Geometry check sheet. Reference: the model listing, model coordinates, mm. A direction names the side the tool comes from. Give positions to 0.01 mm unless a question says otherwise; leave off trailing zeros. Loops run counter-clockwise (first coordinate to the right, second up) from the corner with the lowest first, then second, coordinate; pieces in that order, holes last. Notation, with made-up numbers: (61.25, 18.5) -> (103.25, 18.5) arc R30 cw to (103.25, 48.5) -> close; hole circle Ø5 at (-18, 17). An arc over 180 degrees is marked (long way). Write item = value, one per line. Start each with the question number.
```python
from build123d import *

# Parameters (mm, degrees)
BOSS_EXTRU_1_DEPTH      = 1
ENL_V_MAT_EXTRU_1_DEPTH = 1
BOSS_EXTRU_2_DEPTH      = 5
ESQUISSE4_W             = 8.8
ESQUISSE4_H             = 7.4
ENL_V_MAT_EXTRU_2_DEPTH = 0.5


with BuildPart() as part:
    # Esquisse1 → Boss.-Extru.1 (new body)
    with BuildSketch(Plane.XY):
        with BuildLine():
            Line((-19.325920559, 52.160343492), (-47.644494554, 40.430406076))
            ThreePointArc((-47.644494554, 40.430406076), (-48.617764601, 39.780087822), (-49.268082855, 38.806817776))
            Line((-49.268082855, 38.806817776), (-60.99802027, 10.488243781))
            ThreePointArc((-60.99802027, 10.488243781), (-61.226381673, 9.340193484), (-60.99802027, 8.192143187))
            Line((-60.99802027, 8.192143187), (-49.268082855, -20.126430808))
            ThreePointArc((-49.268082855, -20.126430808), (-48.617764601, -21.099700855), (-47.644494554, -21.750019109))
            Line((-47.644494554, -21.750019109), (-19.325920559, -33.479956525))
            ThreePointArc((-19.325920559, -33.479956525), (-18.177870262, -33.708317927), (-17.029819965, -33.479956525))
            Line((-17.029819965, -33.479956525), (11.28875403, -21.750019109))
            ThreePointArc((11.28875403, -21.750019109), (12.262024077, -21.099700855), (12.912342331, -20.126430808))
            Line((12.912342331, -20.126430808), (24.642279746, 8.192143187))
            ThreePointArc((24.642279746, 8.192143187), (24.870641149, 9.340193484), (24.642279746, 10.488243781))
            Line((24.642279746, 10.488243781), (12.912342331, 38.806817776))
            ThreePointArc((12.912342331, 38.806817776), (12.262024077, 39.780087822), (11.28875403, 40.430406076))
            Line((11.28875403, 40.430406076), (-17.029819965, 52.160343492))
            ThreePointArc((-17.029819965, 52.160343492), (-18.177870262, 52.388704894), (-19.325920559, 52.160343492))
        make_face()
    extrude(amount=BOSS_EXTRU_1_DEPTH)

    # Esquisse2 → Enlèv. mat.-Extru.1 (cut)
    with BuildSketch(Plane.XY.offset(1)):
        with BuildLine():
            Line((-21.671668776, 13.7151444), (-17.371668776, 13.7151444))
            ThreePointArc((-17.371668776, 13.7151444), (-15.271668776, 11.6151444), (-17.371668776, 9.5151444))
            Line((-17.371668776, 9.5151444), (-21.671668776, 9.5151444))
            Line((-21.671668776, 9.5151444), (-21.671668776, 13.7151444))
        make_face()
    extrude(amount=-ENL_V_MAT_EXTRU_1_DEPTH, mode=Mode.SUBTRACT)

    # Esquisse3 → Boss.-Extru.2 (add)
    with BuildSketch(Plane(origin=(0, 0, 0), x_dir=(-1, 0, 0), z_dir=(0, 0, -1))):
        Polygon((47.874104614, 39.036427835), (18.177870262, 51.337010855), (-11.51836409, 39.036427835), (-23.818947109, 9.340193484), (-11.51836409, -20.356040868), (18.177870262, -32.656623888), (47.874104614, -20.356040868), (60.174687633, 9.340193484), align=None)
        Polygon((47.108737749, 38.27106097), (18.177870262, 50.254618655), (-10.752997225, 38.27106097), (-22.736554909, 9.340193484), (-10.752997225, -19.590674003), (18.177870262, -31.574231687), (47.108737749, -19.590674003), (59.092295433, 9.340193484), align=None, mode=Mode.SUBTRACT)
    extrude(amount=BOSS_EXTRU_2_DEPTH)

    # Esquisse4 → Enlèv. mat.-Extru.2 (cut)
    with BuildSketch(Plane(origin=(0, 0, 0), x_dir=(-1, 0, 0), z_dir=(0, 0, -1))):
        with Locations((17.626428794, 11.6151444)):
            Rectangle(ESQUISSE4_W, ESQUISSE4_H)
    extrude(amount=-ENL_V_MAT_EXTRU_2_DEPTH, mode=Mode.SUBTRACT)


solid = part.part
```
1) Draft check along Y on faces 4 (the flat face through (18.695, -6.165, 0.493)), 5 (the flat face through (-19, 1, 0)), 6 (the flat face through (-2.672, 46.213, 0.493)). Enter one of: released by +Y, released by -Y, zero draft, split by the parting line, or undercut.
2) Section check A-A (z = -2.25). Enter the section's corners in (x, y).
3) Section check C-C (x = -39). Enter the section's corners in (y, z), plus the area to 3 significant figures.
4) Section check B-B (y = 20.5). Enter the section's corners in (x, z).
5) Depth check by flat-ended pin: pin 1 Ø8 at (x, y) = (10.5, -14) entering from -Z; pin 2 Ø10 at (x, y) = (-29, 7) entering from -Z; pin 3 Ø1 at (x, z) = (-9, -1.5) entering from +Y. Enter the tip coordinate at first touch or a pass-through.
6) Thickness scan on line 1 (Z direction, x = -36, y = 34); line 2 (X direction, y = 27, z = -2.45); line 3 (X direction, y = 24, z = -1.2). Record the ranges inside material, lowest first.
7) Tool access check on faces 1 (the flat face through (-53.184, 23.603, -2.465)), 2 (the flat face through (-3.12, -26.42, -2.46)), 3 (the flat face through (-33.234, 45.101, -2.465)). Record the directions out of +Z, -Z, +X, -X, +Y, -Y that give a thin tool (end or side, any length) a straight path to the whole face; none if there is none.
Check result:
q1.face_4 = released by -Y
q1.face_5 = undercut
q1.face_6 = released by +Y
q2.outline = (-60.17, 9.34) -> (-47.87, -20.36) -> (-18.18, -32.66) -> (11.52, -20.36) -> (23.82, 9.34) -> (11.52, 39.04) -> (-18.18, 51.34) -> (-47.87, 39.04) -> close; hole (-59.09, 9.34) -> (-47.11, -19.59) -> (-18.18, -31.57) -> (10.75, -19.59) -> (22.74, 9.34) -> (10.75, 38.27) -> (-18.18, 50.25) -> (-47.11, 38.27) -> close
q3.outline = (-25.33, 0) -> (-24.03, 0) -> (-24.03, -5) -> (-22.95, -5) -> (-22.95, 0) -> (41.63, 0) -> (41.63, -5) -> (42.71, -5) -> (42.71, 0) -> (44.01, 0) -> (44.01, 1) -> (-25.33, 1) -> close
q3.area = 80.2 mm2
q4.outline = (-56.85, 0) -> (-55.55, 0) -> (-55.55, -5) -> (-54.47, -5) -> (-54.47, 0) -> (18.11, 0) -> (18.11, -5) -> (19.2, -5) -> (19.2, 0) -> (20.5, 0) -> (20.5, 1) -> (-56.85, 1) -> close
q5.pin_1 = -5
q5.pin_2 = 0
q5.pin_3 = 47.74
q6.line_1 = 0 to 1
q6.line_2 = -52.86 to -51.78, 15.42 to 16.5
q6.line_3 = -54.1 to -53.02, 16.66 to 17.75
q7.face_1 = -Z
q7.face_2 = -Z, +X, -Y
q7.face_3 = -Z, -X, +Y
